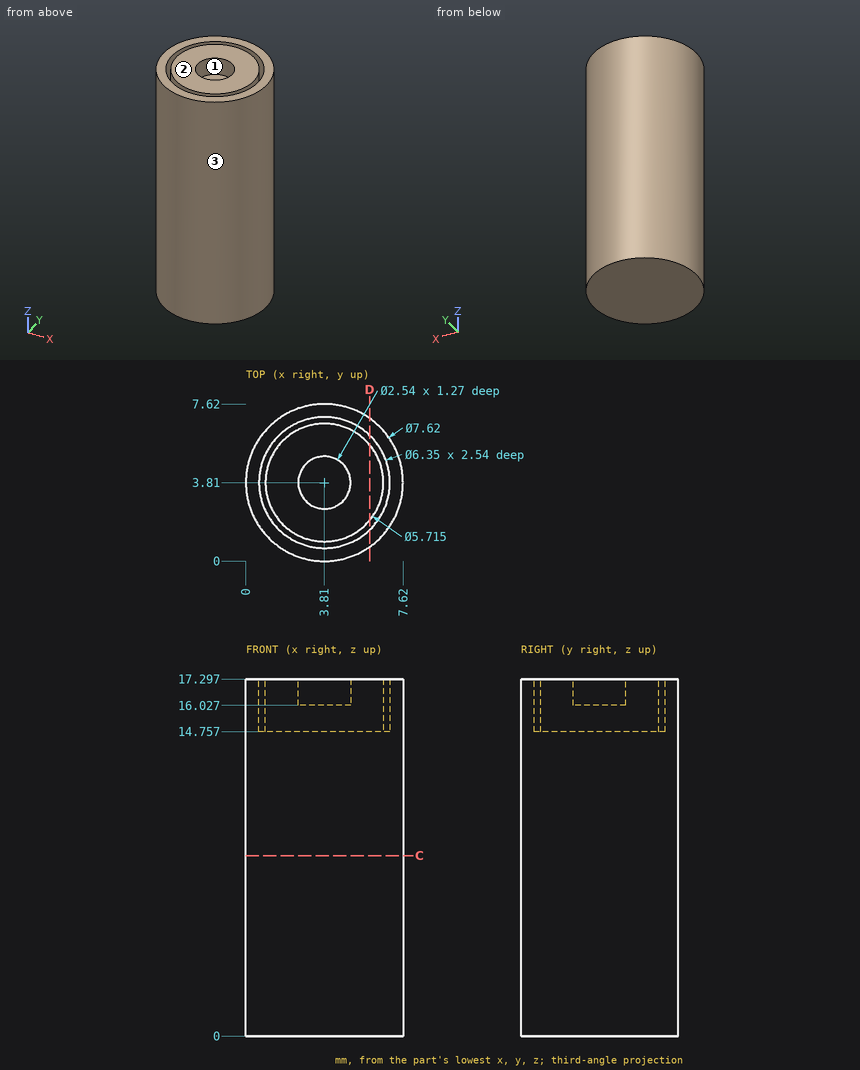
Could you check a few things on this drawing? It's one solid part, dimensions in mm from its lowest x, y, z. Coordinates: 2 decimals unless noted, no trailing zeros. Loops run counter-clockwise (first coordinate to the right, second up) from the corner with the lowest first, then second, coordinate; pieces in that order, holes last. Notation, with made-up numbers: (36.25, 66) - (65.25, 66) arc R11 cw to (65.25, 70) - close; hole circle Ø8 at (-12.5, -29). An arc over 180 degrees is marked (long way). Return JSON: item names as keys, results as strings. Group by question number.
Item 1: If we section it at C-C on z = 8.75: Write out the boundary of the cut face in (x, y).
Item 2: If we section it at D-D on x = 6: Write out the boundary of the cut face in (y, z) (1 decimal).
Item 3: I need wall thicknesses on line 1 (Y direction, x = 3.81, z = 15.45) (1 decimal); line 2 (Y direction, x = 3.81, z = 16.15) (1 decimal); line 3 (Z direction, x = 2.75, y = 6.5). Which ranges of each line are inside material? Lowest first, please. Write a range as from..to.
Item 4: We'd pull the mould along Y, two halves only. Please class the marked faces 1, 2 and 3: +Y half, -Y half, draft (parallel to the pull), parting line (faces both ways), or undercut.
Item 5: Will this pin go through, and if not, where does the flat tip stop? P1, Ø0.8, axis at x = 3.5, y = 4, coming from the +Z side.
Calculated:
{
 "1": {"outline": "circle Ø7.62 at (3.81, 3.81)"},
 "2": {"outline": "(0.7, 0) - (6.9, 0) - (6.9, 17.3) - (6.1, 17.3) - (6.1, 14.8) - (5.6, 14.8) - (5.6, 17.3) - (2, 17.3) - (2, 14.8) - (1.5, 14.8) - (1.5, 17.3) - (0.7, 17.3) - close"},
 "3": {"line 1": "y = 0..0.6, 1..6.7, 7..7.6", "line 2": "y = 0..0.6, 1..2.5, 5.1..6.7, 7..7.6", "line 3": "z = 0..14.76"},
 "4": {"face 1": "undercut", "face 2": "draft", "face 3": "parting line"},
 "5": {"P1": "stops at z = 16.03"}
}
